Check sheet for the modelled part. Datum: model origin and axes. Units: mm. A direction names the side the tool comes from. Coordinates: 2 decimals unless noted, no trailing zeros. Order: outer loops, then holes, each group sorted by start corner. A loop starts at its lowest first (then second) coordinate and runs counter-clockwise, first axis right, second up. Notation, with made-up numbers: (4, -25.75) -> (19, -25.75) arc R32 ccw to (19, 1.25) -> close; hole circle Ø6 at (-18.75, -24.5). An arc over 180 degrees is marked (long way). Put each result on its own line as item: value. Start each with the question number.
```python
from build123d import *

# Parameters (mm, degrees)
SKETCH1_W           = 500
SKETCH1_H           = 150
SKETCH1_R           = 9.3
SKETCH1_R_2         = 3
SKETCH1_R_3         = 4
BOSS_EXTRUDE1_DEPTH = 1.5875
CUT_EXTRUDE1_DEPTH  = 7
SKETCH4_R           = 9.3
CUT_EXTRUDE2_DEPTH  = 10
FILLET1_R           = 2
SKETCH5_R           = 1.75
SKETCH5_R_2         = 1.25
SKETCH5_R_3         = 3
CUT_EXTRUDE3_DEPTH  = 10
SKETCH6_R           = 4
SKETCH6_R_2         = 3
SKETCH6_R_3         = 1.75
CUT_EXTRUDE4_DEPTH  = 10
SKETCH7_R           = 1.75
CUT_EXTRUDE5_DEPTH  = 246.38
SKETCH4_3_R         = 9.3
BOSS_EXTRUDE2_DEPTH = 7.045


with BuildPart() as part:
    # Sketch1 → Boss-Extrude1 (new body)
    with BuildSketch(Plane.XY):
        with Locations((200, 0)):
            Rectangle(SKETCH1_W, SKETCH1_H)
        Circle(SKETCH1_R, mode=Mode.SUBTRACT)
        with BuildLine():
            ThreePointArc((303.594020264, 21.24999987), (340.400100069, 42.5), (377.206179805, 21.249999751))
            ThreePointArc((377.206179805, 21.249999751), (375.559064779, 15.102885357), (369.411950518, 16.750000881))
            ThreePointArc((369.411950518, 16.750000881), (340.40010055, 33.5), (311.388250032, 16.750001833))
            ThreePointArc((311.388250032, 16.750001833), (305.241135638, 15.102885116), (303.594020264, 21.24999987))
        make_face(mode=Mode.SUBTRACT)
        with Locations((376.9688, -9.7841)):
            Circle(SKETCH1_R_2, mode=Mode.SUBTRACT)
        with Locations((340.4001, 0)):
            Circle(SKETCH1_R_3, mode=Mode.SUBTRACT)
    extrude(amount=BOSS_EXTRUDE1_DEPTH)

    # Sketch3 → Cut-Extrude1 (cut)
    with BuildSketch(Plane.XY.offset(1.5875)):
        with BuildLine():
            Line((36.827355724, 55), (-50, 55))
            Line((-50, 55), (-50, -75))
            Line((-50, -75), (450, -75))
            Line((450, -75), (450, 55))
            Line((450, 55), (340.4001, 55))
            ThreePointArc((340.4001, 55), (379.290972965, 38.890872965), (395.4001, 0))
            ThreePointArc((395.4001, 0), (394.567019757, -9.536498518), (392.093016219, -18.7841))
            ThreePointArc((392.093016219, -18.7841), (329.389321669, -53.886573101), (285.481979129, 3))
            Line((285.481979129, 3), (30.896152423, 3))
            Line((30.896152423, 3), (21.172644276, 3))
            Line((21.172644276, 3), (9.086322138, -9.086322138))
            ThreePointArc((9.086322138, -9.086322138), (-9.086322138, -9.086322138), (-9.086322138, 9.086322138))
            Line((-9.086322138, 9.086322138), (36.827355724, 55))
        make_face()
        with BuildLine():
            Line((328.2654389, 3), (285.481979129, 3))
            ThreePointArc((285.481979129, 3), (329.389321669, -53.886573101), (392.093016219, -18.7841))
            Line((392.093016219, -18.7841), (371.332419214, -18.7841))
            Line((371.332419214, -18.7841), (350.803013897, -6.930323401))
            ThreePointArc((350.803013897, -6.930323401), (335.360003988, -11.438856245), (328.2654389, 3))
        make_face()
        Polygon((-50, 75), (-50, 55), (36.827355724, 55), (340.4001, 55), (450, 55), (450, 75), align=None)
    extrude(amount=-CUT_EXTRUDE1_DEPTH, mode=Mode.SUBTRACT)

    # Sketch4 → Cut-Extrude2 (cut)
    with BuildSketch(Plane.XY.offset(1.5875)):
        with BuildLine():
            Line((23.112698372, 8), (6.470027048, 24.642671324))
            Line((6.470027048, 24.642671324), (-9.086322138, 9.086322138))
            ThreePointArc((-9.086322138, 9.086322138), (4.917482106, 11.871851993), (12.85, 0))
            ThreePointArc((12.85, 0), (11.871851993, -4.917482106), (9.086322138, -9.086322138))
            Line((9.086322138, -9.086322138), (21.172644276, 3))
            Line((21.172644276, 3), (41, 3))
            Line((41, 3), (41, 8))
            Line((41, 8), (23.112698372, 8))
        make_face()
        with BuildLine():
            ThreePointArc((12.85, 0), (4.917482106, 11.871851993), (-9.086322138, 9.086322138))
            ThreePointArc((-9.086322138, 9.086322138), (-9.086322138, -9.086322138), (9.086322138, -9.086322138))
            ThreePointArc((9.086322138, -9.086322138), (11.871851993, -4.917482106), (12.85, 0))
        make_face()
        Circle(SKETCH4_R, mode=Mode.SUBTRACT)
        Polygon((36.827355724, 55), (30.827355724, 49), (50.827355724, 49), (50.827355724, 55), align=None)
    extrude(amount=-CUT_EXTRUDE2_DEPTH, mode=Mode.SUBTRACT)

    # Fillet1
    fillet1_edges = [part.edges().sort_by_distance(p)[0] for p in [
        (328.2654389, 3, 0.79375),
        (350.803013897, -6.930323401, 0.79375),
        (392.093016219, -18.7841, 0.79375),
    ]]
    fillet(fillet1_edges, radius=FILLET1_R)

    # Sketch5 → Cut-Extrude3 (cut)
    with BuildSketch(Plane.XY.offset(1.5875)):
        with Locations((17.470027048, 19.642671324)):
            Circle(SKETCH5_R)
        with Locations((42.470027048, 39.642671324)):
            Circle(SKETCH5_R)
        with Locations((93.270027048, 39.642671324)):
            Circle(SKETCH5_R)
        with Locations((68.270027048, 19.642671324)):
            Circle(SKETCH5_R)
        with Locations((119.070027048, 19.642671324)):
            Circle(SKETCH5_R)
        with Locations((75.770027048, 17.642671324)):
            Circle(SKETCH5_R_2)
        with Locations((60.770027048, 17.642671324)):
            Circle(SKETCH5_R_3)
    extrude(amount=-CUT_EXTRUDE3_DEPTH, mode=Mode.SUBTRACT)

    # Sketch6 → Cut-Extrude4 (cut)
    with BuildSketch(Plane.XY.offset(1.5875)):
        with Locations((340.4001, 0)):
            Circle(SKETCH6_R)
        with Locations((376.9688, -9.7841)):
            Circle(SKETCH6_R_2)
        with Locations((350.4001, 7.5)):
            Circle(SKETCH6_R_3)
        with Locations((386.9688, 0)):
            Circle(SKETCH6_R_3)
        with Locations((365.670778247, -10.944141097)):
            Circle(SKETCH6_R_3)
    extrude(amount=-CUT_EXTRUDE4_DEPTH, mode=Mode.SUBTRACT)

    # Sketch7 → Cut-Extrude5 (cut)
    with BuildSketch(Plane.XY.offset(1.5875)):
        with Locations((75.827355724, 49)):
            Circle(SKETCH7_R)
        with Locations((125.827355724, 49)):
            Circle(SKETCH7_R)
        with Locations((175.827355724, 49)):
            Circle(SKETCH7_R)
        with Locations((225.827355724, 49)):
            Circle(SKETCH7_R)
        with Locations((275.827355724, 49)):
            Circle(SKETCH7_R)
        with Locations((325.827355724, 49)):
            Circle(SKETCH7_R)
    extrude(amount=-CUT_EXTRUDE5_DEPTH, mode=Mode.SUBTRACT)

    # Sketch4_3 → Boss-Extrude2 (add)
    with BuildSketch(Plane.XY.offset(1.5875)):
        Polygon((36.827355724, 55), (30.827355724, 49), (50.827355724, 49), (50.827355724, 55), align=None)
        with BuildLine():
            Line((23.112698372, 8), (6.470027048, 24.642671324))
            Line((6.470027048, 24.642671324), (-9.086322138, 9.086322138))
            ThreePointArc((-9.086322138, 9.086322138), (4.917482106, 11.871851993), (12.85, 0))
            ThreePointArc((12.85, 0), (11.871851993, -4.917482106), (9.086322138, -9.086322138))
            Line((9.086322138, -9.086322138), (21.172644276, 3))
            Line((21.172644276, 3), (41, 3))
            Line((41, 3), (41, 8))
            Line((41, 8), (23.112698372, 8))
        make_face()
        with BuildLine():
            ThreePointArc((12.85, 0), (4.917482106, 11.871851993), (-9.086322138, 9.086322138))
            ThreePointArc((-9.086322138, 9.086322138), (-9.086322138, -9.086322138), (9.086322138, -9.086322138))
            ThreePointArc((9.086322138, -9.086322138), (11.871851993, -4.917482106), (12.85, 0))
        make_face()
        Circle(SKETCH4_3_R, mode=Mode.SUBTRACT)
        Polygon((50.827355724, 49), (30.827355724, 49), (6.470027048, 24.642671324), (23.112698372, 8), (41, 8), align=None)
    extrude(amount=-BOSS_EXTRUDE2_DEPTH)


solid = part.part
```
1) Sectioned sample at B-B (x = 204). Record the boundary of the cut face in (y, z), plus the area to 4 significant figures.
2) Mould release check, pull along Y, two halves, no side actions. Record for faces 4 (the flat face through (45.845, 28.213, -2.691)), 5 (the cylindrical face through (-9.284, -8.884, -1.886)), 6 (the cylindrical face through (305.327, 15.054, 0.783)): +Y half, -Y half, draft (parallel to the pull), parting line (faces both ways), or undercut.
3) Sectioned sample at A-A (z = -4). Record the boundary of the cut face in (x, y).
4) Gauge pin test, flat ends, axial feed: pin 1 (16.5 mm diameter, centred on x = 0, y = 0, fed in from -Z); pin 2 (5.5 mm diameter, centred on x = 125.83, y = 49, fed in from -Z); pin 3 (3 mm diameter, centred on y = 22, z = 0.5, fed in from +X). Record the tip position at first contact, or that the pin passes through.
5) Scan lines: line 1 along X through (y, z) = (29.5, 1.25); line 2 along Y through (x, z) = (46, 0.25); line 3 along Z through (x, y) = (234.5, 51.5). Record each from-to range of solid material in increasing order. Write a range as [from, to].
6) Access from +Z, -Z, +X, -X, +Y, -Y to the whole of each face (thin tool, end or side, straight path). Record for faces 1 (the cylindrical face through (339.777, 42.495, 0.783)), 2 (the flat face through (361.96, -13.372, 0.805)), 3 (the flat face through (26, 22, -5.458)).
Entries:
1. outline: (3, 0) -> (55, 0) -> (55, 1.59) -> (3, 1.59) -> close
1. area: 82.55 mm2
2. face 4: -Y half
2. face 5: parting line
2. face 6: undercut
3. outline: (-9.09, 9.09) arc R12.85 ccw to (9.09, -9.09) -> (21.17, 3) -> (41, 3) -> (41, 8) -> (50.83, 49) -> (50.83, 55) -> (36.83, 55) -> close; hole circle Ø18.6 at (0, 0)
4. pin 1: passes through
4. pin 2: stops at z = 0
4. pin 3: stops at x = 391.44
5. line 1: x = [11.33, 309.81], [324.53, 356.27], [370.99, 386.82]
5. line 2: y = [3, 55]
5. line 3: z = [0, 1.59]
6. face 1: +Z, -Z
6. face 2: +Z, -Z, -Y
6. face 3: -Z, +X, -X, +Y, -Y
